```python
from build123d import *

# Parameters (mm, degrees)
F_3_0MM_DOWEL_HOLE1_D        = 3
CUT_EXTRUDE1_DEPTH           = 1.5
CHAMFER1_SIZE                = 1.5
CIRPATTERN1_COUNT            = 3
CHAMFER1_OF_CIRPATTERN1_SIZE = 1.5
CIRPATTERN2_COUNT            = 8


with BuildPart() as part:
    # Sketch1 → Revolve1 (revolve)
    with BuildSketch(Plane.XY):
        with BuildLine():
            Line((16, 0), (25.5, 0))
            Line((25.5, 0), (25.5, 2.5))
            Line((25.5, 2.5), (17.5, 2.5))
            Line((17.5, 2.5), (17.5, 10.3))
            Line((17.5, 10.3), (0, 10.3))
            Line((0, 10.3), (0, 2.5))
            Line((0, 2.5), (0, 0))
            Line((0, 0), (0, -0.8))
            Line((0, -0.8), (0, -6.4))
            Line((0, -6.4), (0, -8.4))
            ThreePointArc((0, -8.4), (0.530330086, -8.619669914), (0.75, -9.15))
            Line((0.75, -9.15), (2, -9.15))
            Line((2, -9.15), (2, -8.9))
            Line((2, -8.9), (7.5, -8.9))
            Line((7.5, -8.9), (7.5, -6.4))
            Line((7.5, -6.4), (12.5, -6.4))
            Line((12.5, -6.4), (12.5, -0.8))
            Line((12.5, -0.8), (16, -0.8))
            Line((16, -0.8), (16, 0))
        make_face()
    revolve(axis=Axis((0, 2.5, 0), (0, 1, 0)))

    # Ø3.0mm Dowel Hole1 (through all)
    with Locations(Plane(origin=(0, 0, 0), x_dir=(-1, 0, 0), z_dir=(0, -1, 0))):
        with Locations((-22, 0)):
            f_3_0mm_dowel_hole1 = Hole(F_3_0MM_DOWEL_HOLE1_D / 2)

    # Sketch5 → Cut-Extrude1 (cut)
    with BuildSketch(Plane.XZ):
        with BuildLine():
            Line((22, -3.5), (25.5, -3.5))
            Line((25.5, -3.5), (25.5, 3.5))
            Line((25.5, 3.5), (22, 3.5))
            ThreePointArc((22, 3.5), (18.5, 0), (22, -3.5))
        make_face()
    cut_extrude1 = extrude(amount=-CUT_EXTRUDE1_DEPTH, mode=Mode.SUBTRACT)

    # Chamfer1
    chamfer1_edges = [part.edges().sort_by_distance(p)[0] for p in [
        (23.62933094, 0, -3.5),
        (18.5, 0, 0),
        (23.62933094, 0, 3.5),
    ]]
    chamfer(chamfer1_edges, length=CHAMFER1_SIZE - 0.0001)  # a hair under: the kernel refuses the full size

    # CirPattern1: Ø3.0mm Dowel Hole1, Cut-Extrude1 ×3 about axis
    cirpattern1_axis = Axis((0, 0, 0), (0, 1, 0))
    add([f_3_0mm_dowel_hole1.rotate(cirpattern1_axis, i * 360 / CIRPATTERN1_COUNT) for i in range(1, CIRPATTERN1_COUNT)], mode=Mode.SUBTRACT)
    add([cut_extrude1.rotate(cirpattern1_axis, i * 360 / CIRPATTERN1_COUNT) for i in range(1, CIRPATTERN1_COUNT)], mode=Mode.SUBTRACT)

    # Chamfer1 of CirPattern1
    chamfer1_of_cirpattern1_edges = [part.edges().sort_by_distance(p)[0] for p in [
        (-14.845754383, 0, -18.713600869),
        (-9.25, 0, -16.02146997),
        (-8.783576557, 0, -22.213600869),
        (-8.783576557, 0, 22.213600869),
        (-9.25, 0, 16.02146997),
        (-14.845754383, 0, 18.713600869),
    ]]
    chamfer(chamfer1_of_cirpattern1_edges, length=CHAMFER1_OF_CIRPATTERN1_SIZE - 0.0001)  # a hair under: the kernel refuses the full size

    # Sketch7 → M2 Tapped Hole1 (revolve, cut)
    with BuildSketch(Plane(origin=(10, -6.4, 0), x_dir=(0, 0, -1), z_dir=(1, 0, 0))):
        Polygon((0, 0), (0, 5.480688495), (0.8, 5), (0.8, 0), align=None)
    m2_tapped_hole1 = revolve(axis=Axis((10, -12.75, 0), (0, 1, 0)), mode=Mode.SUBTRACT)

    # CirPattern2: M2 Tapped Hole1 ×8 about axis
    cirpattern2_axis = Axis((0, 0, 0), (0, 1, 0))
    for i in range(1, CIRPATTERN2_COUNT):
        add(m2_tapped_hole1.rotate(cirpattern2_axis, i * 360 / CIRPATTERN2_COUNT), mode=Mode.SUBTRACT)


solid = part.part
```
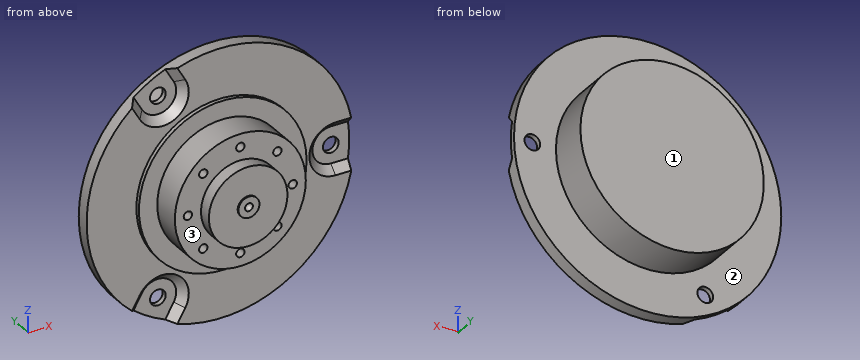
Verification items for the finished model (mm, model axes). Face numbers are marked on the shaded views. A direction names the side the tool comes from. Give positions to 0.01 mm unless a question says otherwise; leave off trailing zeros. Loops run counter-clockwise (first coordinate to the right, second up) from the corner with the lowest first, then second, coordinate; pieces in that order, holes last. Notation, with made-up numbers: M 44.25,-36.75 L 75.25,-36.75 A15 cw 75.25,-29.75 Z; hole C 51.5,-23 d6. An arc over 180 degrees is marked long. Return JSON: item names as keys, results as strings.
1) Material ranges on L1, parallel to Z at x = 0, y = -4.15; L2, parallel to Z at x = 10, y = -3.95, recorded low to high. Write a range as [from, to].
Findings:
{"L1": "z = [-12.5, -10.8], [-9.2, 9.2], [10.8, 12.5]", "L2": "z = [-7.5, -0.8], [0.8, 7.5]"}
2) Section check A-A, the plane y = -5.25. Count the separate pieces of the cut face and the enclosed holes in it, and give its area (3 significant figures).
Findings:
{"separate pieces": "1", "enclosed holes": "8", "area": "475 mm2"}
3) Tool access check on the marked faces 1, 2 and 3. Record the directions out of +Z, -Z, +X, -X, +Y, -Y that give a thin tool (end or side, any length) a straight path to the whole face; none if there is none.
Findings:
{"face 1": "+Z, -Z, +X, -X, +Y", "face 2": "+Y", "face 3": "-Y"}
4) Section check B-B, the plane y = 5.5. Enter the section's corners in (x, z).
Findings:
{"outline": "C 0,0 d35"}
5) Gauge pin test, flat ends, axial feed: P1, Ø2.5, axis at x = 10, z = 0, coming from the -Y side; P2, Ø9.5, axis at x = -1.5, z = 7.5, coming from the -Y side; P3, Ø8, axis at x = 0.5, y = -5, coming from the -Z side. Record the tip position at first contact, or that the pin passes through.
Findings:
{"P1": "stops at y = -6.4", "P2": "stops at y = -8.9", "P3": "stops at z = -12.5"}
6) Section check C-C, the plane x = -20.5. Enter the section's corners in (y, z).
Findings:
{"outline": "M 0,-15.17 L 2.5,-15.17 L 2.5,15.17 L 0,15.17 Z"}
